```python
from build123d import *

# Parameters (mm, degrees)
F0_W     = 16.256
F0_H     = 16.256
F1_DEPTH = 114.3
F0_W_2   = 25.4
F0_H_2   = 25.4
F2_DEPTH = 12.7
F3_R     = 3.048
F4_R     = 12.69999
F0_W_3   = 38.1
F0_H_3   = 38.1
F5_DEPTH = 6.35
F6_R     = 19.04999


# Not quite as in the source:
# - a fillet or chamfer is up to 0.001 mm smaller than in the source, because OpenCascade refuses the exact size


with BuildPart() as f1:
    # F0 (on Top) → F1 (new body)
    with BuildSketch(Plane.XY):
        with Locations((8.128, 8.128)):
            Rectangle(F0_W, F0_H)
    extrude(amount=F1_DEPTH)

    # F0 (on Top) → F2 (join)
    with BuildSketch(Plane.XY):
        with Locations((7.8703831056, 8.128)):
            Rectangle(F0_W_2, F0_H_2)
        with Locations((8.128, 8.128)):
            Rectangle(F0_W, F0_H, mode=Mode.SUBTRACT)
    extrude(amount=F2_DEPTH)

    # F3
    f3_edges = [f1.edges().sort_by_distance(p)[0] for p in [
        (0, 16.256, 63.5),
        (16.256, 16.256, 63.5),
        (16.256, 0, 63.5),
        (0, 0, 63.5),
    ]]
    fillet(f3_edges, radius=F3_R)

    # F4 (radius 12.7 in the source; OpenCascade refuses exactly that, so slightly less here)
    f4_edges = [f1.edges().sort_by_distance(p)[0] for p in [
        (-4.829617, 20.828, 6.35),
        (-4.829617, -4.572, 6.35),
        (20.570383, -4.572, 6.35),
        (20.570383, 20.828, 6.35),
    ]]
    fillet(f4_edges, radius=F4_R)

    # F0 (on Top) → F5 (join)
    with BuildSketch(Plane.XY):
        with Locations((7.8703831056, 8.128)):
            Rectangle(F0_W_3, F0_H_3)
        with Locations((7.8703831056, 8.128)):
            Rectangle(F0_W_2, F0_H_2, mode=Mode.SUBTRACT)
        with Locations((7.8703831056, 8.128)):
            Rectangle(F0_W_2, F0_H_2)
        with Locations((8.128, 8.128)):
            Rectangle(F0_W, F0_H, mode=Mode.SUBTRACT)
    extrude(amount=F5_DEPTH)

    # F6 (radius 19.05 in the source; OpenCascade refuses exactly that, so slightly less here)
    f6_edges = [f1.edges().sort_by_distance(p)[0] for p in [
        (-11.179617, 27.178, 3.175),
        (26.920383, 27.178, 3.175),
        (26.920383, -10.922, 3.175),
        (-11.179617, -10.922, 3.175),
    ]]
    fillet(f6_edges, radius=F6_R)


solid = f1.part
```
Source: CAD feature listing. Evaluate the final solid. Frame: model axes, mm. A direction names the side the tool comes from. Give positions to 0.01 mm unless a question says otherwise; leave off trailing zeros. Loops run counter-clockwise (first coordinate to the right, second up) from the corner with the lowest first, then second, coordinate; pieces in that order, holes last. Notation, with made-up numbers: (56.5, -0.5) -> (91.5, -0.5) arc R20 ccw to (91.5, 33.5) -> close; hole circle Ø9 at (42.25, -25.5). An arc over 180 degrees is marked (long way). Use a Markdown table: item, result. Add a question column.
(1) Section query B-B (y = -2). Output: boundary loops of the cut face in (x, z), then the cut area to 3 significant figures.
(2) First-contact query: pin 1 Ø2 at (y, z) = (12, 21.5) entering from -X; pin 2 Ø6 at (x, y) = (15, -6) entering from +Z; pin 3 Ø1.5 at (y, z) = (4, 32.5) entering from +X. Flat tips, straight axial feed; report the tip coordinate or a pass-through.
(3) Section query D-D (y = 15). Output: boundary loops of the cut face in (x, z).
(4) Section query A-A (z = 40.5). Output: boundary loops of the cut face in (x, y), then the cut area to 3 significant figures.
(5) Ray query, line 1 (X direction, y = 6.5, z = 73); line 2 (Z direction, x = 7.5, y = -8.5). Return the intervals inside material, ascending.
(6) Section query C-C (x = 9). Output: boundary loops of the cut face in (y, z).
(7) Access query for faces 1 (the face through (16.75, -0.95, 9.57)), 2 (the face through (7.7, -0.2, 12.7)), 3 (the face through (0, 8, 63)), 4 (the face through (0.917, 0.869, 64.211)). Directions: +Z, -Z, +X, -X, +Y, -Y. A direction counts if a zero-diameter tool reaches every point of the face in a straight line with its end or side. Return the directions, or none.
Checked values:
| question | item | result |
|---|---|---|
| 1 | outline | (-8.26, 0) -> (24.01, 0) -> (24.01, 6.35) -> (15.53, 6.35) -> (15.53, 12.7) -> (0.21, 12.7) -> (0.21, 6.35) -> (-8.26, 6.35) -> close |
| 1 | area | 302 mm^2 |
| 2 | pin 1 | x = 0 |
| 2 | pin 2 | z = 6.35 |
| 2 | pin 3 | x = 16.26 |
| 3 | outline | (-9.9, 0) -> (25.64, 0) -> (25.64, 6.35) -> (18.55, 6.35) -> (18.55, 12.7) -> (15.67, 12.7) -> (15.67, 114.3) -> (0.58, 114.3) -> (0.58, 12.7) -> (-2.81, 12.7) -> (-2.81, 6.35) -> (-9.9, 6.35) -> close |
| 4 | outline | (0, 3.05) arc R3.05 ccw to (3.05, 0) -> (13.21, 0) arc R3.05 ccw to (16.26, 3.05) -> (16.26, 13.21) arc R3.05 ccw to (13.21, 16.26) -> (3.05, 16.26) arc R3.05 ccw to (0, 13.21) -> close |
| 4 | area | 256 mm^2 |
| 5 | line 1 | 0 to 16.26 |
| 5 | line 2 | 0 to 6.35 |
| 6 | outline | (-10.89, 0) -> (27.14, 0) -> (27.14, 6.35) -> (20.78, 6.35) -> (20.78, 12.7) -> (16.26, 12.7) -> (16.26, 114.3) -> (0, 114.3) -> (0, 12.7) -> (-4.52, 12.7) -> (-4.52, 6.35) -> (-10.89, 6.35) -> close |
| 7 | face 1 | +Z, +X, -Y |
| 7 | face 2 | +Z, +X, -Y |
| 7 | face 3 | +Z, -X, +Y, -Y |
| 7 | face 4 | +Z, -X, -Y |
